Source: three-view drawing plus pictorial views. Frame: mm from the lowest corner of the part. A direction names the side the tool comes from. Give positions to 0.01 mm unless a question says otherwise; leave off trailing zeros. Order: outer loops, then holes, each group sorted by start corner. A loop starts at its lowest first (then second) coordinate and runs counter-clockwise, first axis right, second up.
1) Draft query along Z for the marked faces 1, 2 and 3. Return one class per face: released by +Z, released by -Z, zero draft, split by the parting line, or undercut.
2) Material intervals for line 1 (Z direction, x = 82, y = 42.5); line 2 (Y direction, x = 27, z = 22.5); line 3 (Y direction, x = 42, z = 50) (1 decimal), sorted ascending.
3) Section A-A, the plane y = 36. Return loops of the section in (x, z), plus the area to 3 significant figures.
4) Access query for the marked faces 4 and 5. Directions: +Z, -Z, +X, -X, +Y, -Y. A direction counts if a zero-diameter tool reaches every point of the face in a straight line with its end or side. Return the directions, or none.
5) First-contact query: P1, Ø0.9, axis at y = 61, z = 2, coming from the +X side; P2, Ø0.9, axis at x = 88.5, z = 2, coming from the -Y side; P3, Ø3, axis at x = 23.5, z = 6.5, coming from the +Y side; P4, Ø6, axis at x = 100, y = 42.36, coming from the -Z side. Flat tips, straight axial feed; report the tip coordinate or a pass-through.
6) Section D-D, the plane x = 62.5. Return loops of the section in (y, z) (1 decimal).
7) Section B-B, the plane x = 32.5. Return loops of the section in (y, z) (1 decimal).
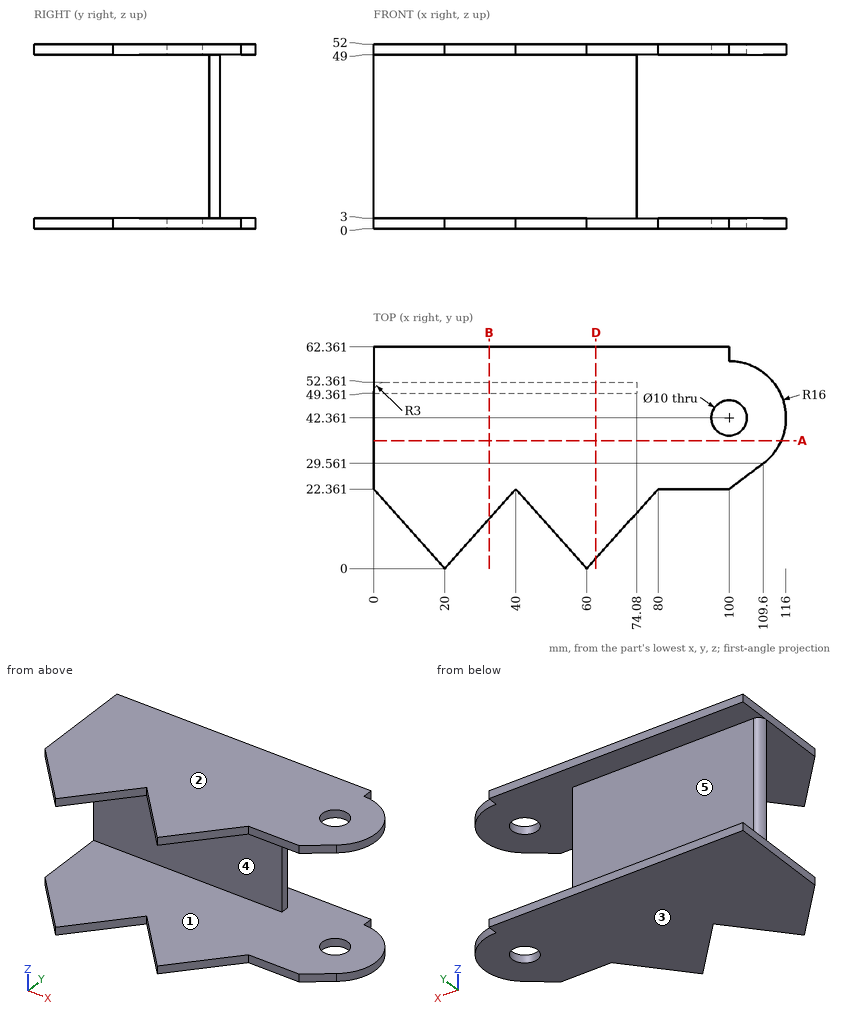
From the geometry:
1. face 1: undercut
1. face 2: released by +Z
1. face 3: released by -Z
2. line 1: z = 0 to 3, 49 to 52
2. line 2: y = 49.36 to 52.36
2. line 3: y = 20.1 to 62.4
3. outline: (0, 0) - (114.68, 0) - (114.68, 3) - (0, 3) - close; (0, 49) - (114.68, 49) - (114.68, 52) - (0, 52) - close
3. area: 688 mm2
4. face 4: +X, -X, -Y
4. face 5: +X, -X, +Y
5. P1: stops at x = 100
5. P2: stops at y = 22.36
5. P3: stops at y = 52.36
5. P4: passes through
6. outline: (2.8, 0) - (62.4, 0) - (62.4, 3) - (52.4, 3) - (52.4, 49) - (62.4, 49) - (62.4, 52) - (2.8, 52) - (2.8, 49) - (49.4, 49) - (49.4, 3) - (2.8, 3) - close
7. outline: (14, 0) - (62.4, 0) - (62.4, 3) - (52.4, 3) - (52.4, 49) - (62.4, 49) - (62.4, 52) - (14, 52) - (14, 49) - (49.4, 49) - (49.4, 3) - (14, 3) - close
